For this review, take the finished solid that the model builds, in its own axes (mm). Face numbers are marked on the shaded views. A direction names the side the tool comes from. Give positions to 0.01 mm unless a question says otherwise; leave off trailing zeros. Write each loop counter-clockwise with the first axis right and the second up, starting at its lowest first coordinate (ties: lowest second). Pieces come first, ordered by that corner, then holes.
1) Machinability: for the marked faces 4 and 5, which of the approach directions +Z, -Z, +X, -X, +Y, -Y give a long, thin tool a straight path to every point of the face, cutting with its end or side? Answer none if there is none.
2) We need section A-A on y = -2.5. Give the boundary of the cut face in (x, z).
3) Wall thickness on line 1 along X through (y, z) = (-2.45, 15.5); line 2 along Z through (x, y) = (15.5, -2.1); line 3 along Y through (x, z) = (-27.5, -44.25): over which ranges is each line inside the solid? List them lowest first.
4) For P1, Ø2, axis at x = 10.5, z = -16.5, coming from the +Y side; P2, Ø4, axis at x = -27.5, y = 3.5, coming from the -Z side; P3, Ø1.8, axis at x = -27, y = 3, coming from the -Z side, all flat-tipped, find the tip position at first contact; note any pin that passes through.
5) We need section C-C on x = 0. Give the boundary of the cut face in (y, z).
6) Draft analysis for pull direction Z (two halves, no side actions). For the marked faces 1, 2 and 3, state which applies: pulls with the +Z half, pulls with the -Z half, needs draft (parallel to the pull), parting line crosses it, or undercut.
7) We need section D-D on x = 15.5. Give the number of separate pieces and of enclosed holes in the cut face, and give its area (3 significant figures).
8) We need section B-B on z = 0. Give the boundary of the cut face in (x, y), and give its area (3 significant figures).
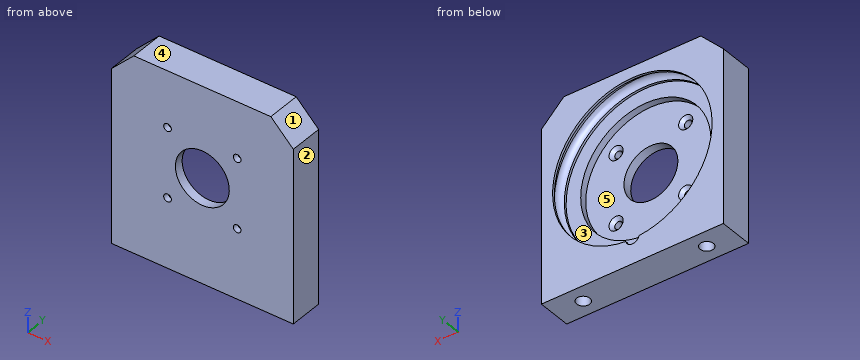
from build123d import *

# Parameters (mm, degrees)
SKETCH3_R                                           = 1.25
CUT_EXTRUDE1_DEPTH                                  = 59.322379924
SKETCH5_R                                           = 3.05
SKETCH6_R                                           = 3
CUT_EXTRUDE2_DEPTH                                  = 10
BOSS_EXTRUDE1_START                                 = -15
BOSS_EXTRUDE1_DEPTH                                 = 15
CHAMFER1_SIZE                                       = 10
CSK_FOR_M3_COUNTERSUNK_FLAT_HEAD_SCREW1_D           = 3.4
CSK_FOR_M3_COUNTERSUNK_FLAT_HEAD_SCREW1_CSINK_D     = 6.3
CSK_FOR_M3_COUNTERSUNK_FLAT_HEAD_SCREW1_CSINK_ANGLE = 90
SKETCH15_W                                          = 81
SKETCH15_H                                          = 15
BOSS_EXTRUDE2_DEPTH                                 = 6
SKETCH16_R                                          = 2.95
CUT_EXTRUDE3_DEPTH                                  = 6.8
M4_CLEARANCE_HOLE1_D                                = 4.8
M4_CLEARANCE_HOLE1_DEPTH                            = 14
M4_CLEARANCE_HOLE1_TIP                              = 1.442065486


with BuildPart() as part:
    # Sketch2 → Revolve1 (revolve)
    with BuildSketch(Plane.XY, mode=Mode.PRIVATE) as revolve1_sk:
        Polygon((-29, 3), (-29, 0), (-12, 0), (-12, -4), (-40.5, -4), (-40.5, 11), (-35.5, 11), (-35.5, 3), align=None)
    revolve(revolve1_sk.sketch.rotate(Axis((0, 0, 0), (0, 1, 0)), 270), axis=Axis((0, 0, 0), (0, 1, 0)))

    # Sketch3 → Cut-Extrude1 (cut, through all)
    with BuildSketch(Plane(origin=(0, 0, 0), x_dir=(1, 0, 0), z_dir=(0, 1, 0))):
        with Locations(Location((-15.5, 15.5, 0), (0, 0, 270))):
            Circle(SKETCH3_R)
        with Locations(Location((15.5, 15.5, 0), (0, 0, 270))):
            Circle(SKETCH3_R)
        with Locations(Location((15.5, -15.5, 0), (0, 0, 270))):
            Circle(SKETCH3_R)
        with Locations(Location((-15.5, -15.5, 0), (0, 0, 270))):
            Circle(SKETCH3_R)
    extrude(amount=-CUT_EXTRUDE1_DEPTH, mode=Mode.SUBTRACT)

    # Sketch5 → Cut-Revolve1 (revolve, cut)
    with BuildSketch(Plane.XY, mode=Mode.PRIVATE) as cut_revolve1_sk:
        with Locations((34.75, 7)):
            Circle(SKETCH5_R)
    revolve(cut_revolve1_sk.sketch.rotate(Axis((0, 0, 0), (0, -1, 0)), 270), axis=Axis((0, 0, 0), (0, -1, 0)), mode=Mode.SUBTRACT)

    # Sketch6 → Cut-Extrude2 (cut)
    with BuildSketch(Plane(origin=(0, 7, 0), x_dir=(1, 0, 0), z_dir=(0, 1, 0))):
        with Locations((0, 34.75)):
            Circle(SKETCH6_R)
    extrude(amount=CUT_EXTRUDE2_DEPTH, mode=Mode.SUBTRACT)

    # Sketch8 → Boss-Extrude1 (add)
    with BuildSketch(Plane.XZ.offset(4).offset(BOSS_EXTRUDE1_START)):
        with BuildLine():
            Line((-40.5, 1.41e-07), (-40.5, -40.5))
            Line((-40.5, -40.5), (-8.3e-08, -40.5))
            ThreePointArc((-8.3e-08, -40.5), (-28.637824717, -28.637824559), (-40.5, 1.41e-07))
        make_face()
        with BuildLine():
            ThreePointArc((40.5, 0), (28.637824609, -28.637824667), (-8.3e-08, -40.5))
            Line((-8.3e-08, -40.5), (40.5, -40.5))
            Line((40.5, -40.5), (40.5, 0))
        make_face()
        with BuildLine():
            Line((-40.5, 40.5), (-40.5, 1.41e-07))
            ThreePointArc((-40.5, 1.41e-07), (-28.637824588, 28.637824688), (0, 40.5))
            Line((0, 40.5), (-40.5, 40.5))
        make_face()
        with BuildLine():
            ThreePointArc((0, 40.5), (28.637824638, 28.637824638), (40.5, 0))
            Line((40.5, 0), (40.5, 40.5))
            Line((40.5, 40.5), (0, 40.5))
        make_face()
    extrude(amount=BOSS_EXTRUDE1_DEPTH)

    # Chamfer1
    chamfer1_edges = [part.edges().sort_by_distance(p)[0] for p in [
        (-40.5, 3.5, 40.5),
        (40.5, 3.5, 40.5),
    ]]
    chamfer(chamfer1_edges, length=CHAMFER1_SIZE)

    # CSK for M3 Countersunk Flat Head Screw1 (through all)
    with Locations(Plane(origin=(0, 0, 0), x_dir=(1, 0, 0), z_dir=(0, 1, 0))):
        with Locations((-15.5, 15.5), (15.5, 15.5), (15.5, -15.5), (-15.5, -15.5)):
            CounterSinkHole(CSK_FOR_M3_COUNTERSUNK_FLAT_HEAD_SCREW1_D / 2, CSK_FOR_M3_COUNTERSUNK_FLAT_HEAD_SCREW1_CSINK_D / 2, counter_sink_angle=CSK_FOR_M3_COUNTERSUNK_FLAT_HEAD_SCREW1_CSINK_ANGLE)

    # Sketch15 → Boss-Extrude2 (add)
    with BuildSketch(Plane(origin=(0, 0, -40.5), x_dir=(-1, 0, 0), z_dir=(0, 0, -1))):
        with Locations((0, 3.5)):
            Rectangle(SKETCH15_W, SKETCH15_H)
    extrude(amount=BOSS_EXTRUDE2_DEPTH)

    # Sketch16 → Cut-Extrude3 (cut)
    with BuildSketch(Plane(origin=(0, 0, -46.5), x_dir=(-1, 0, 0), z_dir=(0, 0, -1))):
        with Locations((-27.5, 3.5)):
            Circle(SKETCH16_R)
        with Locations(Location((27.5, 3.5, 0), (0, 0, 180))):
            Circle(SKETCH16_R)
    extrude(amount=-CUT_EXTRUDE3_DEPTH, mode=Mode.SUBTRACT)

    # M4 Clearance Hole1
    with Locations(Plane(origin=(0, 0, -46.5), x_dir=(-1, 0, 0), z_dir=(0, 0, -1))):
        with Locations((-27.5, 3.5), (27.5, 3.5)):
            Hole(M4_CLEARANCE_HOLE1_D / 2, depth=M4_CLEARANCE_HOLE1_DEPTH)
            with Locations((0, 0, -(M4_CLEARANCE_HOLE1_DEPTH + M4_CLEARANCE_HOLE1_TIP / 2))):  # 118° drill point
                Cone(0, M4_CLEARANCE_HOLE1_D / 2, M4_CLEARANCE_HOLE1_TIP, mode=Mode.SUBTRACT)


solid = part.part
Results list:
1. face 4: +Z, +X, -X, +Y, -Y
1. face 5: +Y
2. outline: (-40.5, -46.5) - (40.5, -46.5) - (40.5, 30.5) - (30.5, 40.5) - (-30.5, 40.5) - (-40.5, 30.5) - close; hole circle Ø3.4 at (-15.5, -15.5); hole circle Ø3.4 at (-15.5, 15.5); hole circle Ø24 at (0, 0); hole circle Ø3.4 at (15.5, -15.5); hole circle Ø3.4 at (15.5, 15.5)
3. line 1: x = -40.5 to -17.2, -13.8 to 13.8, 17.2 to 40.5
3. line 2: z = -46.5 to -17.2, -13.8 to 13.8, 17.2 to 40.5
3. line 3: y = -4 to 0.55, 6.45 to 11
4. P1: stops at y = 0
4. P2: stops at z = -32.26
4. P3: stops at z = -32.02
5. outline: (-4, -46.5) - (11, -46.5) - (11, -37.75) - (7.55, -37.75) arc R3.05 cw to (4.04, -35.5) - (3, -35.5) - (3, -29) - (0, -29) - (0, -12) - (-4, -12) - close; (-4, 12) - (0, 12) - (0, 29) - (3, 29) - (3, 35.5) - (4.04, 35.5) arc R3.05 cw to (9.96, 35.5) - (11, 35.5) - (11, 40.5) - (-4, 40.5) - close
6. face 1: pulls with the +Z half
6. face 2: needs draft
6. face 3: undercut
7. separate pieces: 3
7. enclosed holes: 0
7. area: 593 mm2
8. outline: (-40.5, -4) - (-12, -4) - (-12, 0) - (-29, 0) - (-29, 3) - (-35.5, 3) - (-35.5, 4.04) arc R3.05 cw to (-35.5, 9.96) - (-35.5, 11) - (-40.5, 11) - close; (12, -4) - (40.5, -4) - (40.5, 11) - (35.5, 11) - (35.5, 9.96) arc R3.05 cw to (35.5, 4.04) - (35.5, 3) - (29, 3) - (29, 0) - (12, 0) - close
8. area: 357 mm2
